Autodesk Inventor part; units mm, degrees
ref_plane "YZ Plane" through (0, 0, 0) normal (1, 0, 0) x (0, 1, 0)
ref_plane "XZ Plane" through (0, 0, 0) normal (0, 1, 0) x (-1, 0, 0)
ref_plane "XY Plane" through (0, 0, 0) normal (0, 0, 1) x (1, 0, 0)
sketch "Esboço1" plane through (0, 0, 0) normal (0, 1, 0) x (-1, 0, 0)
  circle A0 centre (0, 0) radius 2.8
  dimension "d0" = 5.6
extrude "Extrusão1" add sketch "Esboço1" along normal blind 2.4
sketch "Esboço2" plane through (0, 0, 0) normal (1, 0, 0) x (0, 1, 0)
  line L0 (0, 0.9185) -> (1.2961, 0.9185)
  line L1 (1.2961, 0.9185) -> (1.2961, -0.9611)
  line L2 (1.2961, -0.9611) -> (0, -0.9611)
  line L3 (0, -0.9611) -> (0, 0.9185)
  point P0 (0, 0)
extrude "Extrusão2" cut sketch "Esboço2" along normal through all both and the other way through all
sketch "Esboço3" plane through (0, 2.4, 0) normal (0, 1, 0) x (1, 0, 0)
  circle A0 centre (0, 0) radius 2.8
  circle A1 centre (0, 0) radius 1.5
  dimension "d5" = 3
extrude "Extrusão3" add sketch "Esboço3" along normal blind 8.5 contours A1
thread "Rosca1"
properties part number "Parafuso-M3-8.5"
Check sheet for the modelled part. Datum: model origin and axes. Units: mm. A direction names the side the tool comes from. Give positions to 0.01 mm unless a question says otherwise; leave off trailing zeros. Write each loop counter-clockwise with the first axis right and the second up, starting at its lowest first coordinate (ties: lowest second). Pieces come first, ordered by that corner, then holes.
Item 1: Access from +Z, -Z, +X, -X, +Y, -Y to the whole of each face (thin tool, end or side, straight path). Record for faces 1 (the face through (0, 1, 0.918)), 2 (the face through (0, 10.9, 0)).
Item 2: Cross-section at D-D (x = -2.4). Enter the section's corners in (y, z), and give its area (3 significant figures).
Item 3: Draft check along Z on faces 3 (the face through (-1.5, 6.59, 0.07)), 4 (the face through (0, 1, -0.961)), 5 (the face through (-1.2, 2.4, -1.2)). Enter one of: released by +Z, released by -Z, zero draft, split by the parting line, or undercut.
Item 4: Scan lines: L1, parallel to Y at x = 1.95, z = -0.55; L2, parallel to Y at x = 0.9, z = 2.15; L3, parallel to Z at x = 0.4, y = 2.75. Record each from-to range of solid material in increasing order.
Item 5: Cross-section at C-C (y = 1.5). Enter the section's corners in (x, z), and give its area (3 significant figures).
Item 6: Cross-section at B-B (z = 0). Enter the section's corners in (x, y), and give its area (3 significant figures).
Item 7: Gauge pin test, flat ends, axial feed: pin 1 (3 mm diameter, centred on x = 0, y = 6.5, fed in from -Z); pin 2 (0.6 mm diameter, centred on x = 1.5, z = 0, fed in from -Y); pin 3 (1.7 mm diameter, centred on x = 1.5, z = 1.5, fed in from +Y). Record the tip position at first contact, or that the pin passes through.
Item 8: Cross-section at A-A (x = 0). Enter the section's corners in (y, z).
Report:
1. face 1: +X, -X, -Y
1. face 2: +Z, -Z, +X, -X, +Y
2. outline: (0, -1.44) - (2.4, -1.44) - (2.4, 1.44) - (0, 1.44) - (0, 0.92) - (1.3, 0.92) - (1.3, -0.96) - (0, -0.96) - close
2. area: 4.49 mm2
3. face 3: split by the parting line
3. face 4: undercut
3. face 5: zero draft
4. L1: y = 1.3 to 2.4
4. L2: y = 0 to 2.4
4. L3: z = -1.45 to 1.45
5. outline: circle Ø5.6 at (0, 0)
5. area: 24.6 mm2
6. outline: (-2.8, 1.3) - (2.8, 1.3) - (2.8, 2.4) - (1.5, 2.4) - (1.5, 10.9) - (-1.5, 10.9) - (-1.5, 2.4) - (-2.8, 2.4) - close
6. area: 31.7 mm2
7. pin 1: stops at z = -1.5
7. pin 2: stops at y = 1.3
7. pin 3: stops at y = 10.9
8. outline: (0, -2.8) - (2.4, -2.8) - (2.4, -1.5) - (10.9, -1.5) - (10.9, 1.5) - (2.4, 1.5) - (2.4, 2.8) - (0, 2.8) - (0, 0.92) - (1.3, 0.92) - (1.3, -0.96) - (0, -0.96) - close
